```python
from build123d import *

# Parameters (mm, degrees)
F0_R     = 27.5
F2_DEPTH = 2
F1_R     = 10.5
F3_DEPTH = 60
F4_R     = 27.5
F5_DEPTH = 2
F6_R     = 9.5
F7_DEPTH = 64


with BuildPart() as f2:
    # F0 (on Top) → F2 (new body)
    with BuildSketch(Plane.XY):
        Circle(F0_R)
    extrude(amount=F2_DEPTH)

    # F1 (on Top) → F3 (join)
    with BuildSketch(Plane.XY):
        Circle(F1_R)
    extrude(amount=-F3_DEPTH)

    # F4 (on face) → F5 (join)
    with BuildSketch(Plane(origin=(0, 0, -60), x_dir=(1, 0, 0), z_dir=(0, 0, -1))):
        Circle(F4_R)
    extrude(amount=F5_DEPTH)

    # F6 (on face) → F7 (cut, through all)
    with BuildSketch(Plane.XY.offset(2)):
        Circle(F6_R)
    extrude(amount=-F7_DEPTH, mode=Mode.SUBTRACT)


solid = f2.part
```
Design review of the part built by this model. Coordinates are the model's own, in mm. A direction names the side the tool comes from. Coordinates: 2 decimals unless noted, no trailing zeros. Loops run counter-clockwise (first coordinate to the right, second up) from the corner with the lowest first, then second, coordinate; pieces in that order, holes last. Notation, with made-up numbers: (50, 46.5) -> (80, 46.5) arc R17 ccw to (80, 77.5) -> close; hole circle Ø3 at (21.5, 87). An arc over 180 degrees is marked (long way). Answer as a JSON object with one key per item and string values.
Q1. The part is to be moulded in two halves that separate along Z. For faces 1 (the flat face through (0, -12, 0)), 2 (the flat face through (0, 12, -60)), 3 (the cylindrical face through (4.38, -8.43, -29.55)), 4 (the flat face through (0, -12, 2)), say which applies: +Z half, -Z half, draft (parallel to the pull), parting line (faces both ways), or undercut.
Answer block:
{"face 1": "undercut", "face 2": "undercut", "face 3": "draft", "face 4": "+Z half"}
Q2. Take a section at D-D on z = -25. Give the boundary of the cut face in (x, y), plus the area to 3 significant figures.
Answer block:
{"outline": "circle Ø21 at (0, 0); hole circle Ø19 at (0, 0)", "area": "62.8 mm^2"}
Q3. Tool access review of faces 5 (the cylindrical face through (-5.961, -26.846, 0.986)), 6 (the cylindrical face through (10, 3.2, -29.6)): name each direction out of +Z, -Z, +X, -X, +Y, -Y from which nothing blocks a thin tool from reaching the whole face with its end or side.
Answer block:
{"face 5": "+Z, -Z", "face 6": "none"}
Q4. To check wall thickness, follow L1, parallel to Z at x = 13, y = 16; L2, parallel to Y at x = 0, z = -29; L3, parallel to X at y = -0.5, z = -57.5. State the ranges of each line that lie inside material, in increasing order.
Answer block:
{"L1": "z = -62 to -60, 0 to 2", "L2": "y = -10.5 to -9.5, 9.5 to 10.5", "L3": "x = -10.49 to -9.49, 9.49 to 10.49"}
Q5. Take a section at B-B on x = 0. Give the boundary of the cut face in (y, z), plus the area to 3 significant figures.
Answer block:
{"outline": "(-27.5, -62) -> (-9.5, -62) -> (-9.5, 2) -> (-27.5, 2) -> (-27.5, 0) -> (-10.5, 0) -> (-10.5, -60) -> (-27.5, -60) -> close; (9.5, -62) -> (27.5, -62) -> (27.5, -60) -> (10.5, -60) -> (10.5, 0) -> (27.5, 0) -> (27.5, 2) -> (9.5, 2) -> close", "area": "264 mm^2"}
Q6. Take a section at A-A on y = 22. Give the boundary of the cut face in (x, z).
Answer block:
{"outline": "(-16.5, -62) -> (16.5, -62) -> (16.5, -60) -> (-16.5, -60) -> close; (-16.5, 0) -> (16.5, 0) -> (16.5, 2) -> (-16.5, 2) -> close"}
Q7. Clearance check with flat-ended pins moving along their axes: pin 1 Ø2 at (x, z) = (-10.5, -51.5) entering from -Y; pin 2 Ø8 at (y, z) = (7, -44) entering from -X; pin 3 Ø12 at (x, z) = (-5, -33) entering from +Y; pin 4 Ø2 at (x, z) = (-12, -10) entering from +Y. State where each tip first meets the part, or that it passes through.
Answer block:
{"pin 1": "stops at y = -4.47", "pin 2": "stops at x = -10.06", "pin 3": "stops at y = 10.5", "pin 4": "passes through"}
